Design review of the part built by this model. Coordinates are the model's own, in mm. Face numbers are marked on the shaded views. A direction names the side the tool comes from. Coordinates: 2 decimals unless noted, no trailing zeros. Write each loop counter-clockwise with the first axis right and the second up, starting at its lowest first coordinate (ties: lowest second). Pieces come first, ordered by that corner, then holes.
Q1. Take a section at D-D (y = 28.27). Give the boundary of the cut face in (x, z).
Q2. Machinability: for the marked faces 4, 5 and 6, which of the approach directions +Z, -Z, +X, -X, +Y, -Y give a long, thin tool a straight path to every point of the face, cutting with its end or side? Answer none if there is none.
Q3. For probe 1 along X at (y, z) = (8, 8.75); probe 2 along X at (y, z) = (12.5, 7); probe 3 along Y at (x, z) = (-53.2, 5.5), list the stretches that pass through material, from the lowest coordinate up.
Q4. Take a section at C-C (x = -46.5). Give the boundary of the cut face in (y, z).
Q5. Take a section at A-A (y = 0). Give the boundary of the cut face in (x, z).
Q6. Take a section at B-B (y = 8). Give the boundary of the cut face in (x, z), and give its area (3 significant figures).
Q7. Insertion check: pin 1 (3.5 mm diameter, centred on x = -8.5, z = 6, fed in from -Y); pin 2 (2.5 mm diameter, centred on x = -54, z = 7, fed in from -Y); pin 3 (8 mm diameter, centred on x = -17.5, y = 25, fed in from -Z); pin 4 (4 mm diameter, centred on y = 28.27, z = 5.5, fed in from +X). Each pin has a flat end and moves straight along its axis. Give the tip position at first contact, or say it passes through.
Q8. Mouldability with a two-part tool opening along X and no side actions: class the marked faces 1, 2 and 3 as pulls with the +X half, pulls with the -X half, needs draft (parallel to the pull), parting line crosses it, or undercut.
```python
from build123d import *

# Parameters (mm, degrees)
BOSS_EXTRUDE1_DEPTH = 10
CUT_EXTRUDE1_REACH  = 86.489
SKETCH2_R           = 1.5
FILLET3_R           = 5
CUT_EXTRUDE2_REACH  = 86.489
SKETCH3_R           = 1.5
FILLET4_R           = 25
CUT_EXTRUDE7_DEPTH  = 1
FILLET8_R           = 0.3
SKETCH8_W           = 10
SKETCH8_H           = 20.75
BOSS_EXTRUDE2_DEPTH = 1
SKETCH10_W          = 4
SKETCH10_H          = 22
CUT_EXTRUDE9_DEPTH  = 1.5
FILLET10_R          = 40


with BuildPart() as part:
    # Sketch1 → Boss-Extrude1 (new body)
    with BuildSketch(Plane.XY):
        with BuildLine():
            Line((13.02, -7.9417418), (17.7, -7.9417418))
            Line((17.7, -7.9417418), (17.7, 38.77))
            Line((17.7, 38.77), (-56.7, 38.77))
            Line((-56.7, 38.77), (-56.7, -6.23))
            Line((-56.7, -6.23), (-51.7, -6.23))
            Line((-51.7, -6.23), (-51.7, 33.77))
            Line((-51.7, 33.77), (-10.566443095, 33.77))
            Line((-10.566443095, 33.77), (-10.566443095, 13.02))
            Line((-10.566443095, 13.02), (-5.317126718, 13.02))
            Line((-5.317126718, 13.02), (-4.287512407, 13.02))
            ThreePointArc((-4.287512407, 13.02), (-3.319474451, 12.619025549), (-2.9185, 11.650987593))
            Line((-2.9185, 11.650987593), (-2.9185, 11.539212407))
            ThreePointArc((-2.9185, 11.539212407), (-3.319474451, 10.571174451), (-4.287512407, 10.1702))
            Line((-4.287512407, 10.1702), (-6.476788598, 10.1702))
            ThreePointArc((-6.476788598, 10.1702), (-7.136510935, 9.729114651), (-6.981020848, 8.950903446))
            Line((-6.981020848, 8.950903446), (-3.672257405, 5.649701928))
            ThreePointArc((-3.672257405, 5.649701928), (-2.746830644, 5.032499411), (-1.655778399, 4.8158))
            Line((-1.655778399, 4.8158), (1.655778399, 4.8158))
            ThreePointArc((1.655778399, 4.8158), (2.746830644, 5.032499411), (3.672257405, 5.649701928))
            Line((3.672257405, 5.649701928), (6.981020848, 8.950903446))
            ThreePointArc((6.981020848, 8.950903446), (7.136510935, 9.729114651), (6.476788598, 10.1702))
            Line((6.476788598, 10.1702), (4.287512407, 10.1702))
            ThreePointArc((4.287512407, 10.1702), (3.319474451, 10.571174451), (2.9185, 11.539212407))
            Line((2.9185, 11.539212407), (2.9185, 11.650987593))
            ThreePointArc((2.9185, 11.650987593), (3.319474451, 12.619025549), (4.287512407, 13.02))
            Line((4.287512407, 13.02), (6.332886163, 13.02))
            Line((6.332886163, 13.02), (10.562594215, 13.019824354))
            ThreePointArc((10.562594215, 13.019824354), (12.303594776, 12.313982883), (13.019956614, 10.577284622))
            Line((13.019956614, 10.577284622), (13.02, 4.287469289))
            ThreePointArc((13.02, 4.287469289), (12.619025549, 3.319431332), (11.650987593, 2.918456882))
            Line((11.650987593, 2.918456882), (11.539212407, 2.918456882))
            ThreePointArc((11.539212407, 2.918456882), (10.571174451, 3.319431332), (10.1702, 4.287469289))
            Line((10.1702, 4.287469289), (10.1702, 6.402089023))
            ThreePointArc((10.1702, 6.402089023), (9.733877283, 7.055496588), (8.963146507, 6.90287605))
            Line((8.963146507, 6.90287605), (5.667020993, 3.614283579))
            ThreePointArc((5.667020993, 3.614283579), (5.046449321, 2.687255303), (4.8285, 1.593185507))
            Line((4.8285, 1.593185507), (4.8285, -1.593185507))
            ThreePointArc((4.8285, -1.593185507), (5.046449321, -2.687255303), (5.667020993, -3.614283579))
            Line((5.667020993, -3.614283579), (8.963146507, -6.90287605))
            ThreePointArc((8.963146507, -6.90287605), (9.733877283, -7.055496588), (10.1702, -6.402089023))
            Line((10.1702, -6.402089023), (10.1702, -4.287469289))
            ThreePointArc((10.1702, -4.287469289), (10.571174451, -3.319431332), (11.539212407, -2.918456882))
            Line((11.539212407, -2.918456882), (11.650987593, -2.918456882))
            ThreePointArc((11.650987593, -2.918456882), (12.619025549, -3.319431332), (13.02, -4.287469289))
            Line((13.02, -4.287469289), (13.02, -5.3170836))
            Line((13.02, -5.3170836), (13.02, -7.9417418))
        make_face()
    extrude(amount=BOSS_EXTRUDE1_DEPTH)

    # Sketch2 → Cut-Extrude1 (cut, up to next)
    with BuildSketch(Plane.ZY.offset(56.7), mode=Mode.PRIVATE) as cut_extrude1_sk1:
        with Locations((5.5, -2.73)):
            Circle(SKETCH2_R)
    cut_extrude1_tool1 = extrude(cut_extrude1_sk1.sketch, amount=-CUT_EXTRUDE1_REACH, mode=Mode.PRIVATE) & part.part
    # Sketch2 → Cut-Extrude1 (cut, up to next)
    with BuildSketch(Plane.ZY.offset(56.7), mode=Mode.PRIVATE) as cut_extrude1_sk2:
        with Locations((5.5, 28.27)):
            Circle(SKETCH2_R)
    cut_extrude1_tool2 = extrude(cut_extrude1_sk2.sketch, amount=-CUT_EXTRUDE1_REACH, mode=Mode.PRIVATE) & part.part
    add(cut_extrude1_tool1.solids().sort_by_distance((-56.7, -2.73, 5.5))[0], mode=Mode.SUBTRACT)
    add(cut_extrude1_tool2.solids().sort_by_distance((-56.7, 28.27, 5.5))[0], mode=Mode.SUBTRACT)

    # Fillet3
    fillet3_edges = [part.edges().sort_by_distance(p)[0] for p in [
        (-56.7, 38.77, 5),
    ]]
    fillet(fillet3_edges, radius=FILLET3_R)

    # Sketch3 → Cut-Extrude2 (cut, up to next)
    with BuildSketch(Plane(origin=(17.7, 0, 0), x_dir=(0, 0, -1), z_dir=(1, 0, 0)), mode=Mode.PRIVATE) as cut_extrude2_sk1:
        with Locations((-7.25, 0)):
            Circle(SKETCH3_R)
    cut_extrude2_tool1 = extrude(cut_extrude2_sk1.sketch, amount=-CUT_EXTRUDE2_REACH, mode=Mode.PRIVATE) & part.part
    # Sketch3 → Cut-Extrude2 (cut, up to next)
    with BuildSketch(Plane(origin=(17.7, 0, 0), x_dir=(0, 0, -1), z_dir=(1, 0, 0)), mode=Mode.PRIVATE) as cut_extrude2_sk2:
        with Locations(Location((-2.75, 0, 0), (0, 0, 90))):
            Circle(SKETCH3_R)
    cut_extrude2_tool2 = extrude(cut_extrude2_sk2.sketch, amount=-CUT_EXTRUDE2_REACH, mode=Mode.PRIVATE) & part.part
    add(cut_extrude2_tool1.solids().sort_by_distance((17.7, 0, 7.25))[0], mode=Mode.SUBTRACT)
    add(cut_extrude2_tool2.solids().sort_by_distance((17.7, 0, 2.75))[0], mode=Mode.SUBTRACT)

    # Fillet4
    fillet4_edges = [part.edges().sort_by_distance(p)[0] for p in [
        (17.7, 38.77, 5),
    ]]
    fillet(fillet4_edges, radius=FILLET4_R)

    # Sketch7 → Cut-Extrude7 (cut)
    with BuildSketch(Plane.XY.offset(10)):
        Polygon((-0.90100078, 19.84300121), (-0.90100078, 27.034293528), (0.113155829, 27.034293528), (0.113155829, 20.672765708), (3.524409877, 20.672765708), (3.524409877, 19.84300121), align=None)
    extrude(amount=-CUT_EXTRUDE7_DEPTH, mode=Mode.SUBTRACT)

    # Fillet8
    fillet8_edges = [part.edges().sort_by_distance(p)[0] for p in [
        (1.311704549, 19.84300121, 10),
        (-0.90100078, 23.438647369, 10),
        (-0.393922475, 27.034293528, 10),
        (0.113155829, 23.853529618, 10),
        (1.818782853, 20.672765708, 10),
        (3.524409877, 20.257883459, 10),
        (1.311704549, 19.84300121, 9),
        (-0.90100078, 23.438647369, 9),
        (-0.393922475, 27.034293528, 9),
        (0.113155829, 23.853529618, 9),
        (1.818782853, 20.672765708, 9),
        (3.524409877, 20.257883459, 9),
    ]]
    fillet(fillet8_edges, radius=FILLET8_R)

    # Sketch8 → Boss-Extrude2 (add)
    with BuildSketch(Plane.ZY.offset(10.566443095)):
        with Locations((5, 23.395)):
            Rectangle(SKETCH8_W, SKETCH8_H)
    extrude(amount=BOSS_EXTRUDE2_DEPTH)

    # Sketch10 → Cut-Extrude9 (cut)
    with BuildSketch(Plane(origin=(0, 0, 0), x_dir=(-1, 0, 0), z_dir=(0, 0, -1))):
        with Locations((51.7, 12.77)):
            Rectangle(SKETCH10_W, SKETCH10_H)
    extrude(amount=-CUT_EXTRUDE9_DEPTH, mode=Mode.SUBTRACT)

    # Fillet10
    # the kernel refuses this fillet: 40 mm, written as the material it adds along each edge
    with BuildSketch(Plane(origin=(-51.7, 1.77, 1.5), x_dir=(0, 0, -1), z_dir=(-1, 0, 0))) as fillet10_piece_1:
        with BuildLine():
            CenterArc((40, -10.851267207), FILLET10_R, 164.259451475, 15.740548525)
            Line((0, -10.851267207), (0, 0))
            Line((0, 0), (1.5, 0))
        make_face()
    extrude(amount=2)
    with BuildSketch(Plane(origin=(-53.7, 23.77, 1.5), x_dir=(0, -1, 0), z_dir=(1, 0, 0))) as fillet10_piece_2:
        with BuildLine():
            CenterArc((10.851267207, 40), FILLET10_R, 254.259451475, 15.740548525)
            Line((0, 1.5), (0, 0))
            Line((0, 0), (10.851267207, 0))
        make_face()
    extrude(amount=2)


solid = part.part
```
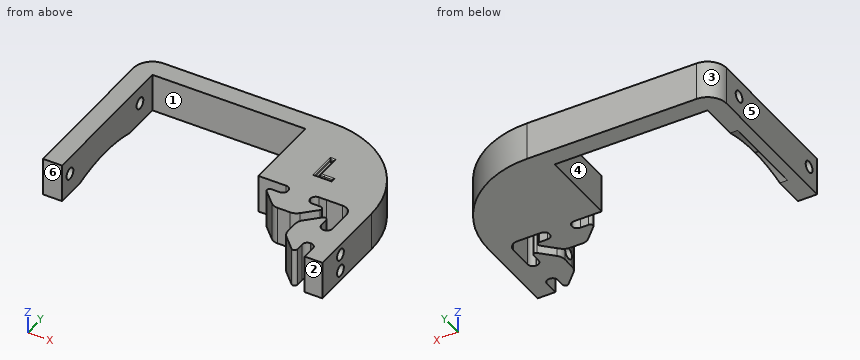
Response:
1. outline: (-56.7, 0) - (-51.7, 0) - (-51.7, 4) - (-56.7, 4) - close; (-56.7, 7) - (-51.7, 7) - (-51.7, 10) - (-56.7, 10) - close; (-11.57, 0) - (13.07, 0) - (13.07, 10) - (-11.57, 10) - close
2. face 4: +Z, -Z, -Y
2. face 5: +Z, -Z, -X, +Y, -Y
2. face 6: +Z, -Z, -X, -Y
3. probe 1: x = -56.7 to -51.7, -6.03 to 6.03, 13.02 to 17.7
3. probe 2: x = -56.7 to -51.7, -3.21 to 3.21, 12.09 to 17.7
3. probe 3: y = -6.23 to -4.23, -1.23 to 26.77, 29.77 to 38.54
4. outline: (33.77, 0) - (38.77, 0) - (38.77, 10) - (33.77, 10) - close
5. outline: (-56.7, 0) - (-51.7, 0) - (-51.7, 10) - (-56.7, 10) - close; (4.83, 0) - (17.7, 0) - (17.7, 1.25) - (4.83, 1.25) - close; (4.83, 4.25) - (17.7, 4.25) - (17.7, 5.75) - (4.83, 5.75) - close; (4.83, 8.75) - (17.7, 8.75) - (17.7, 10) - (4.83, 10) - close
6. outline: (-56.7, 0) - (-53.7, 0) - (-53.7, 1.23) - (-51.7, 1.23) - (-51.7, 10) - (-56.7, 10) - close; (-6.03, 0) - (6.03, 0) - (6.03, 10) - (-6.03, 10) - close; (13.02, 0) - (17.7, 0) - (17.7, 10) - (13.02, 10) - close
6. area: 215 mm2
7. pin 1: stops at y = 8.72
7. pin 2: stops at y = -6.23
7. pin 3: passes through
7. pin 4: stops at x = 14.35
8. face 1: undercut
8. face 2: needs draft
8. face 3: pulls with the -X half
